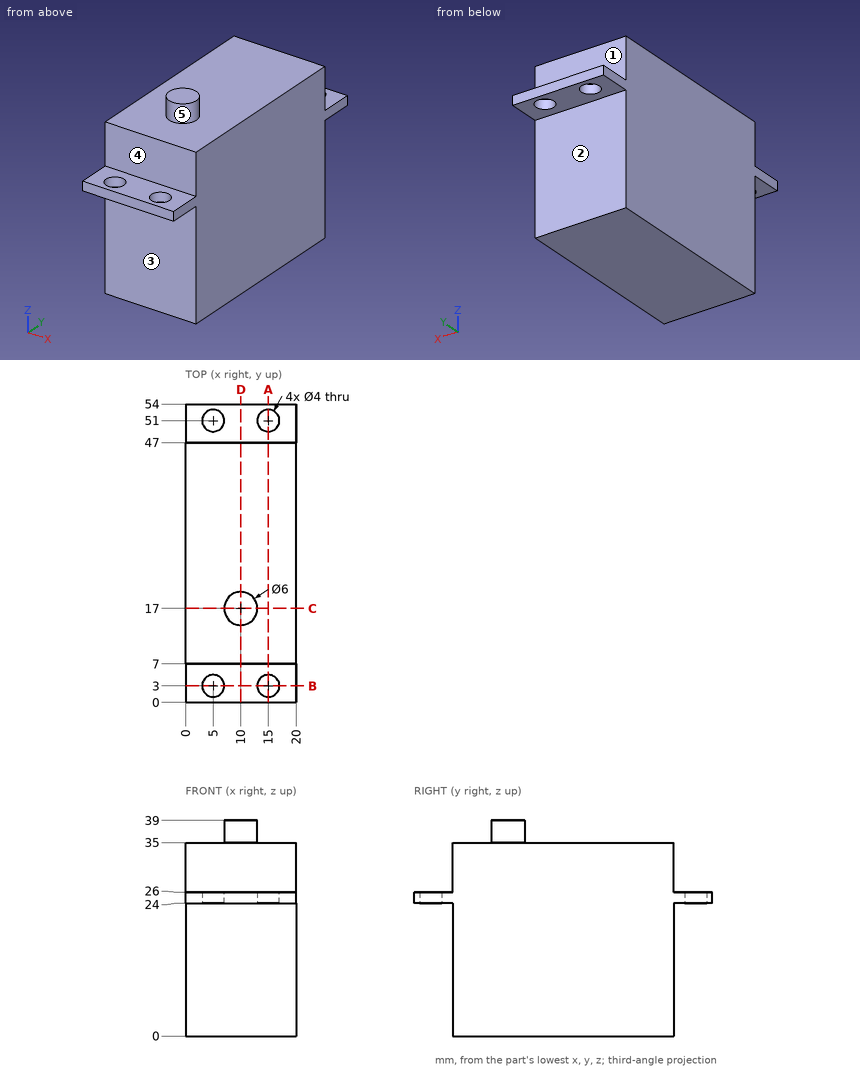
Study the drawing (mm; zero at the part's minimum x, y, z) and answer. A direction names the side the tool comes from. Coordinates: 2 decimals unless noted, no trailing zeros. Write each loop counter-clockwise with the first axis right and the second up, starting at its lowest first coordinate (ties: lowest second). Pieces come first, ordered by that corner, then holes.
Q1. Section C-C, the plane y = 17 is taken. Write down the section's boundary in (x, z), then the cut area to 3 significant figures.
Returned:
outline: (0, 0) - (20, 0) - (20, 35) - (13, 35) - (13, 39) - (7, 39) - (7, 35) - (0, 35) - close
area: 724 mm2
Q2. Given P1, Ø7.5, axis at x = 14.5, y = 3, coming from the +Z side; P2, Ø10, axis at x = 14.5, z = 16, coming from the -Y side; P3, Ø6, axis at x = 13.5, y = 11.5, coming from the +Z side, each flat-ended and moving along its own axis, determine where each tip first touches the part or whether it passes through.
Returned:
P1: stops at z = 26
P2: stops at y = 7
P3: stops at z = 35
Q3. Find the intervals of material crossed by line 1 along Y through (x, z) = (5, 24.5); line 2 along Z through (x, y) = (6.5, 37); line 3 along Y through (x, z) = (15, 7), in increasing order.
Returned:
line 1: y = 0 to 1, 5 to 49, 53 to 54
line 2: z = 0 to 35
line 3: y = 7 to 47
Q4. Section B-B, the plane y = 3 is taken. Write down the section's boundary in (x, z).
Returned:
outline: (0, 24) - (3, 24) - (3, 26) - (0, 26) - close; (7, 24) - (13, 24) - (13, 26) - (7, 26) - close; (17, 24) - (20, 24) - (20, 26) - (17, 26) - close
Q5. Section A-A, the plane x = 15 is taken. Write down the section's boundary in (y, z).
Returned:
outline: (0, 24) - (1, 24) - (1, 26) - (0, 26) - close; (5, 24) - (7, 24) - (7, 0) - (47, 0) - (47, 24) - (49, 24) - (49, 26) - (47, 26) - (47, 35) - (7, 35) - (7, 26) - (5, 26) - close; (53, 24) - (54, 24) - (54, 26) - (53, 26) - close
Q6. Which of the six approach directions +Z, -Z, +X, -X, +Y, -Y give full straight-line access (tool end or side, diameter ignored) to the marked faces 1, 2, 3, 4 and 5?
Returned:
face 1: +Z, +X, -X, +Y
face 2: -Z, +X, -X, +Y
face 3: -Z, +X, -X, -Y
face 4: +Z, +X, -X, -Y
face 5: +Z
Q7. Section D-D, the plane x = 10 is taken. Write down the section's boundary in (y, z), then the cut area to 3 significant figures.
Returned:
outline: (0, 24) - (7, 24) - (7, 0) - (47, 0) - (47, 24) - (54, 24) - (54, 26) - (47, 26) - (47, 35) - (20, 35) - (20, 39) - (14, 39) - (14, 35) - (7, 35) - (7, 26) - (0, 26) - close
area: 1,450 mm2
